Could you check a few things on this model? Use its own coordinates, in mm. A direction names the side the tool comes from. Coordinates: 2 decimals unless noted, no trailing zeros. Write each loop counter-clockwise with the first axis right and the second up, starting at its lowest first coordinate (ties: lowest second). Pieces come first, ordered by that corner, then holes. Notation, with made-up numbers: M -10,9.25 L -2,9.25 A19 ccw -2,40.25 Z; hole C 15.25,31.25 d2. An arc over 180 degrees is marked long. Answer as CSV lines item,"result". Start each with the question number.
Item 1: Suppose I cut it at C-C, the plane x = 3. Write out the boundary of the cut face in (y, z), and give its area (3 significant figures).
Item 2: Suppose I cut it at A-A, the plane z = -50. Write out the boundary of the cut face in (x, y).
Item 3: Suppose I cut it at B-B, the plane y = 15.25. Write out the boundary of the cut face in (x, z) (3 decimals), and give its area (3 significant figures).
Item 4: On a 3-axis mill with a long thin cutter (end or side, diameter ignored), from which of +Z, -Z, +X, -X, +Y, -Y can I reach the whole of each face in a straight line? I mean faces 1 (the flat face through (-11, 10, -1.495)), 2 (the flat face through (22.5, 10, 2)). Say none if no direction works.
Item 5: If I drill on line 1 along Z through (x, y) = (9.5, 3.75); line 2 along Z through (x, y) = (11.5, 13.5); line 3 along Z through (x, y) = (-7.5, 14.25) (3 decimals), over which ranges is the centre line in solid material (lowest first)? Write a range as [from, to].
Item 6: Suppose I cut it at D-D, the plane z = 106. Write out the boundary of the cut face in (x, y).
Autodesk Inventor part; units mm, degrees
ref_plane "YZ Plane" through (0, 0, 0) normal (1, 0, 0) x (0, 1, 0)
ref_plane "XZ Plane" through (0, 0, 0) normal (0, 1, 0) x (-1, 0, 0)
ref_plane "XY Plane" through (0, 0, 0) normal (0, 0, 1) x (1, 0, 0)
sketch "Sketch1" plane through (0, 0, 0) normal (0, 1, 0) x (-1, 0, 0)
  line L0 (22.5, 125) -> (-22.5, 125)
  line L1 (-22.5, 125) -> (-22.5, -125)
  line L2 (-22.5, -125) -> (22.5, -125)
  line L3 (22.5, -125) -> (22.5, 125)
  line L4 (22.5, 125) -> (-22.5, -125) construction
  line L5 (-22.5, 125) -> (22.5, -125) construction
  point P0 (0, 0)
  dimension "d0" = 250
  dimension "d1" = 45
extrude "Extrusion1" add sketch "Sketch1" along normal blind 20
sketch "Sketch2" plane through (0, 0, 0) normal (0, -1, 0) x (1, 0, 0)
  circle A0 centre (0, 100) radius 17.75
  circle A1 centre (0, 50) radius 17.75
  circle A2 centre (0, -50) radius 17.75
  line L0 (0, 50) -> (0, -50) construction
  line L1 (0, 100) -> (0, 50) construction
  line L2 (0, 0) -> (0, 148) construction
  line L3 (-35.7491, 0) -> (26.8031, 0) construction
  line L4 (0, -1.495) -> (-22.5, -1.495)
  line L5 (-22.5, -1.495) -> (-22.5, 1.495)
  line L6 (-22.5, 1.495) -> (0, 1.495)
  line L7 (0, 1.495) -> (0, -1.495)
  line L8 (0, -1.495) -> (-22.5, 1.495) construction
  line L9 (-22.5, -1.495) -> (0, 1.495) construction
  line L10 (-18, 98) -> (-18, -100)
  line L11 (-22.5, 125) -> (22.5, 125)
  line L12 (-22.5, -125) -> (-22.5, 125)
  point P0 (0, 75)
  point P1 (-11.5, 0)
  point P2 (-11.25, 0)
  point P3 (-25, -148)
  point P4 (-16, 100)
  dimension "d9" = 35.5
  dimension "d10" = 35.5
  dimension "d11" = 35.5
  dimension "d12" = 50
  dimension "d13" = 100
  dimension "d16" = 2.99
  dimension "d36" = 25
extrude "Extrusion5" cut sketch "Sketch2" against normal through all
equation "\"d9\" = d11"
equation "\"d10\" = d11"
equation "\"d13\" = 2 * d12"
properties part number "stand3" material "Wood (Walnut)"
Ans:
1,outline,"M 0,-125 L 20,-125 L 20,-67.49 L 0,-67.49 Z; M 0,-32.51 L 20,-32.51 L 20,32.51 L 0,32.51 Z; M 0,67.49 L 20,67.49 L 20,82.51 L 0,82.51 Z; M 0,117.49 L 20,117.49 L 20,125 L 0,125 Z"
1,area,"2,900 mm^2"
2,outline,"M -22.5,0 L -17.75,0 L -17.75,20 L -22.5,20 Z; M 17.75,0 L 22.5,0 L 22.5,20 L 17.75,20 Z"
3,outline,"M -22.5,-125 L 22.5,-125 L 22.5,125 L -22.5,125 L -22.5,1.495 L 0,1.495 L 0,-1.495 L -22.5,-1.495 Z; hole C 0,-50 d35.5; hole C 0,50 d35.5; hole C 0,100 d35.5"
3,area,"8,210 mm^2"
4,face 1,"-X, +Y, -Y"
4,face 2,"+Z, -Z, +X, +Y, -Y"
5,line 1,"z = [-125, -64.99], [-35.01, 35.01], [64.99, 85.01], [114.99, 125]"
5,line 2,"z = [-125, -63.52], [-36.48, 36.48], [63.52, 86.48], [113.52, 125]"
5,line 3,"z = [-125, -66.088], [-33.912, -1.495], [1.495, 33.912], [66.088, 83.912], [116.088, 125]"
6,outline,"M -22.5,0 L -16.71,0 L -16.71,20 L -22.5,20 Z; M 16.71,0 L 22.5,0 L 22.5,20 L 16.71,20 Z"
